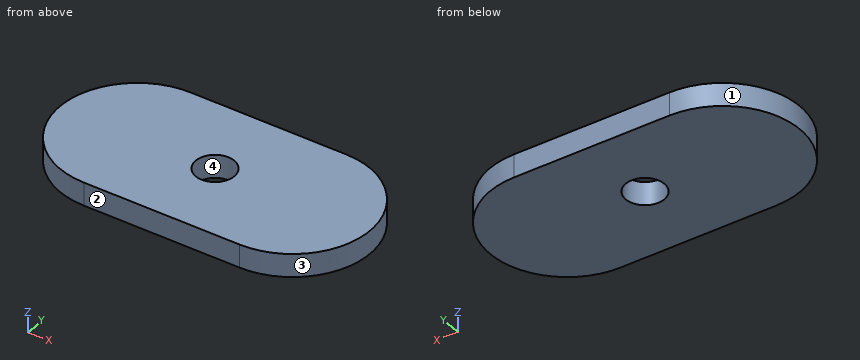
```python
from build123d import *

# Parameters (mm, degrees)
F0_W     = 20
F0_H     = 20
F0_R     = 2.5
F1_DEPTH = 3


with BuildPart() as f1:
    # F0 (on Top) → F1 (new body)
    with BuildSketch(Plane.XY):
        with BuildLine():
            ThreePointArc((-10, 10), (-20, 0), (-10, -10))
            Line((-10, -10), (-10, 10))
        make_face()
        Rectangle(F0_W, F0_H)
        Circle(F0_R, mode=Mode.SUBTRACT)
        with BuildLine():
            Line((10, 10), (10, -10))
            ThreePointArc((10, -10), (20, 0), (10, 10))
        make_face()
    extrude(amount=F1_DEPTH)


solid = f1.part
```
The listing builds one solid part. Answer for the finished solid, in the listing's coordinates (mm). Face numbers are marked on the shaded views. Give positions to 0.01 mm unless a question says otherwise; leave off trailing zeros. Order: outer loops, then holes, each group sorted by start corner. A loop starts at its lowest first (then second) coordinate and runs counter-clockwise, first axis right, second up. Notation, with made-up numbers: (63, 75.5) -> (94, 75.5) arc R15 ccw to (94, 103.5) -> close; hole circle Ø6 at (83.5, 13.25). An arc over 180 degrees is marked (long way). One line per item, written item: value.
1) Find section A-A, the plane x = 0. Determine the outline of the cut face in (y, z).
Reported:
outline: (-10, 0) -> (-2.5, 0) -> (-2.5, 3) -> (-10, 3) -> close; (2.5, 0) -> (10, 0) -> (10, 3) -> (2.5, 3) -> close
2) Find section C-C, the plane y = 0. Determine the outline of the cut face in (x, z).
Reported:
outline: (-20, 0) -> (-2.5, 0) -> (-2.5, 3) -> (-20, 3) -> close; (2.5, 0) -> (20, 0) -> (20, 3) -> (2.5, 3) -> close
3) Find section D-D, the plane y = -7. Determine the outline of the cut face in (x, z).
Reported:
outline: (-17.14, 0) -> (17.14, 0) -> (17.14, 3) -> (-17.14, 3) -> close
4) Determine the mould class of the marked faces 1, 2, 3 and 4 for opening direction X: pulls with the +X half, pulls with the -X half, needs draft (parallel to the pull), parting line crosses it, or undercut.
Reported:
face 1: pulls with the -X half
face 2: needs draft
face 3: pulls with the +X half
face 4: undercut
5) Find the intervals of material crossed by line 1 (Y direction, x = 0, z = 1.5); line 2 (Y direction, x = -2, z = 0.3); line 3 (X direction, y = -6.75, z = 0.7), in increasing order.
Reported:
line 1: y = -10 to -2.5, 2.5 to 10
line 2: y = -10 to -1.5, 1.5 to 10
line 3: x = -17.38 to 17.38
6) Find section B-B, the plane z = 0.4. Determine the outline of the cut face in (x, y), plus the area to 3 significant figures.
Reported:
outline: (-10, -10) -> (10, -10) arc R10 ccw to (10, 10) -> (-10, 10) arc R10 ccw to start; hole circle Ø5 at (0, 0)
area: 695 mm^2
